```python
from build123d import *

# Parameters (mm, degrees)
SKETCH_1_R        = 4.5
SKETCH_1_R_2      = 3
EXTRUDE_1_DEPTH   = 1.9
SKETCH_1_R_3      = 4
SKETCH_1_R_4      = 2.5
EXTRUDE_1_2_DEPTH = 1.9
EXTRUDE_START     = -1.9
EXTRUDE_2_DEPTH   = 1.9
FILLET_1_R        = 10
FILLET_2_R        = 5


with BuildPart() as part:
    # Sketch 1 → Extrude 1 (new body)
    with BuildSketch(Plane.XY):
        with Locations(Location((35, 0, 0), (0, 0, 180))):
            Circle(SKETCH_1_R)
        with Locations(Location((35, 0, 0), (0, 0, 180))):
            Circle(SKETCH_1_R_2, mode=Mode.SUBTRACT)
    extrude(amount=EXTRUDE_1_DEPTH)



with BuildPart() as body_2:
    # Sketch 1 → Extrude 1 2 (new body)
    with BuildSketch(Plane.XY):
        with Locations(Location((0, 0, 0), (0, 0, 180))):
            Circle(SKETCH_1_R_3)
        with Locations(Location((0, 0, 0), (0, 0, 180))):
            Circle(SKETCH_1_R_4, mode=Mode.SUBTRACT)
    extrude(amount=EXTRUDE_1_2_DEPTH)


with BuildPart() as part_1:
    add(part.part)

    add(body_2.part)  # Extrude 2 merges body 2
    # Sketch 3 → Extrude 2 (add)
    with BuildSketch(Plane.XY.offset(1.9).offset(EXTRUDE_START)):
        with BuildLine():
            Line((30.505314037, -0.218627753), (22.960861135, -4.430337969))
            Line((22.960861135, -4.430337969), (3.878251034, 0.979371696))
            ThreePointArc((3.878251034, 0.979371696), (3.848349766, -1.090964748), (2.787286286, -2.868978069))
            Line((2.787286286, -2.868978069), (23.463935052, -8.730580129))
            Line((23.463935052, -8.730580129), (32.455079681, -3.71125054))
            ThreePointArc((32.455079681, -3.71125054), (31.070799365, -2.19348635), (30.505314037, -0.218627753))
        make_face()
    extrude(amount=EXTRUDE_2_DEPTH)

    # Fillet 1
    fillet_1_edges = [part_1.edges().sort_by_distance(p)[0] for p in [
        (22.960861135, -4.430337969, 0.95),
        (23.463935052, -8.730580129, 0.95),
    ]]
    fillet(fillet_1_edges, radius=FILLET_1_R)

    # Fillet 2
    fillet_2_edges = [part_1.edges().sort_by_distance(p)[0] for p in [
        (3.878251034, 0.979371696, 0.95),
        (30.505314037, -0.218627753, 0.95),
        (32.455079681, -3.71125054, 0.95),
        (2.787286286, -2.868978069, 0.95),
    ]]
    fillet(fillet_2_edges, radius=FILLET_2_R)


solid = part_1.part
```
CAD build for the part. Positions are in the model's coordinates, mm. A direction names the side the tool comes from. Round coordinates to 2 decimals unless told otherwise and drop trailing zeros. Loops run counter-clockwise (first coordinate to the right, second up) from the corner with the lowest first, then second, coordinate; pieces in that order, holes last. Notation, with made-up numbers: M -21,9.25 L 16,9.25 A34 cw 16,45.25 Z; hole C -2.75,53.5 d3. An arc over 180 degrees is marked long. Return JSON: item names as keys, results as strings. Group by question number.
(1) Drop a flat-ended pin along its axis: P1, Ø5, axis at x = 35, y = 0, coming from the +Z side. Give the stop position or say it passes through.
(2) Saw through at B-B, the plane z = 1.5. List the corners of the cut face in (x, y), and give its area (3 significant figures).
(3) Saw through at A-A, the plane x = 0. List the corners of the cut face in (y, z).
(4) Tool access for faces 5 (the cylindrical face through (38, 0, 1)), 6 (the flat face through (12.573, -1.485, 0.937)): list every direction of +Z, -Z, +X, -X, +Y, -Y with a clear straight run to the whole face (end or side of a thin tool).
(5) Saw through at D-D, the plane x = 34.5. List the corners of the cut face in (y, z).
(6) Mould opens along X. For faces 1 (the flat face through (18.05, -3.21, 0)), 2 (the cylindrical face through (38.998, 2.065, 0.937)), 3 (the cylindrical face through (23.31, -7.92, 0.96)), 4 (the flat face through (27.51, -1.89, 0.94)) say: +X half, -X half, draft (parallel to the pull), parting line (faces both ways), or undercut.
(7) Saw through at C-C, the plane y = 0. List the corners of the cut face in (x, z).
(8) Wall check: probe 1 along Y at (x, z) = (0, 1.2); probe 2 along Y at (x, z) = (35, 1.1); probe 3 along X at (y, z) = (1.25, 1.1). Give the ranges that are in metal, low to high. Write a range as [from, to].
Answer list:
{
 "1": {"P1": "through"},
 "2": {"outline": "M 1.57,-3.68 A5 cw 4.9,-3.47 L 19.48,-7.6 A10 ccw 27.08,-6.71 L 30.37,-4.88 A5 cw 33.96,-4.38 A4.5 ccw long 30.73,1.41 A5 cw 28.42,-1.38 L 26.58,-2.41 A10 cw 18.98,-3.3 L 5.99,0.38 A5 cw 3.27,2.31 A4 ccw long Z; hole C 0,0 d5; hole C 35,0 d6", "area": "186 mm2"},
 "3": {"outline": "M -4,0 L -2.5,0 L -2.5,1.9 L -4,1.9 Z; M 2.5,0 L 4,0 L 4,1.9 L 2.5,1.9 Z"},
 "4": {"face 5": "+Z, -Z", "face 6": "+Z, -Z, +Y"},
 "5": {"outline": "M -4.47,0 L -2.96,0 L -2.96,1.9 L -4.47,1.9 Z; M 2.96,0 L 4.47,0 L 4.47,1.9 L 2.96,1.9 Z"},
 "6": {"face 1": "draft", "face 2": "undercut", "face 3": "parting line", "face 4": "undercut"},
 "7": {"outline": "M -4,0 L -2.5,0 L -2.5,1.9 L -4,1.9 Z; M 2.5,0 L 7.33,0 L 7.33,1.9 L 2.5,1.9 Z; M 29.99,0 L 32,0 L 32,1.9 L 29.99,1.9 Z; M 38,0 L 39.5,0 L 39.5,1.9 L 38,1.9 Z"},
 "8": {"probe 1": "[-4, -2.5], [2.5, 4]", "probe 2": "[-4.5, -3], [3, 4.5]", "probe 3": "[-3.8, -2.17], [2.17, 4.28], [30.67, 32.27], [37.73, 39.32]"}
}
